```python
from build123d import *

# Parameters (mm, degrees)
SKETCH_1_W          = 17
SKETCH_1_H          = 11.5
EXTRUDE_1_DEPTH     = 1.5
SKETCH_2_R          = 4
EXTRUDE_2_DEPTH     = 3
SKETCH_3_R          = 2
CUT_EXTRUDE_1_DEPTH = 0.2
SKETCH_4_R          = 0.5
SKETCH_4_R_2        = 1.5
CUT_EXTRUDE_2_DEPTH = 11.69170239


with BuildPart() as part:
    # Эскиз1 → Бобышка-Вытянуть1 (new body)
    with BuildSketch(Plane(origin=(0, 0, 0), x_dir=(1, 0, 0), z_dir=(0, 1, 0))):
        Rectangle(SKETCH_1_W, SKETCH_1_H)
    extrude(amount=EXTRUDE_1_DEPTH)

    # Эскиз2 → Бобышка-Вытянуть2 (add)
    with BuildSketch(Plane(origin=(0, 1.5, 0), x_dir=(1, 0, 0), z_dir=(0, 1, 0))):
        with Locations(Location((0, 0, 0), (0, 0, 270))):
            Circle(SKETCH_2_R)
    extrude(amount=EXTRUDE_2_DEPTH)

    # Эскиз3 → Вырез-Вытянуть1 (cut)
    with BuildSketch(Plane(origin=(0, 4.5, 0), x_dir=(1, 0, 0), z_dir=(0, 1, 0))):
        with Locations(Location((0, 0, 0), (0, 0, 270))):
            Circle(SKETCH_3_R)
    extrude(amount=-CUT_EXTRUDE_1_DEPTH, mode=Mode.SUBTRACT)

    # Эскиз4 → Вырез-Вытянуть2 (cut, through all)
    with BuildSketch(Plane(origin=(0, 1.5, 0), x_dir=(1, 0, 0), z_dir=(0, 1, 0))):
        with Locations(Location((6.5, 3.81, 0), (0, 0, 270))):
            Circle(SKETCH_4_R)
        with Locations(Location((6.5, 1.27, 0), (0, 0, 270))):
            Circle(SKETCH_4_R)
        with Locations(Location((6.5, -1.27, 0), (0, 0, 270))):
            Circle(SKETCH_4_R)
        with Locations(Location((6.5, -3.81, 0), (0, 0, 270))):
            Circle(SKETCH_4_R)
        with Locations(Location((-6.43732089, 3, 0), (0, 0, 270))):
            Circle(SKETCH_4_R_2)
        with Locations(Location((-6.43732089, -3, 0), (0, 0, 270))):
            Circle(SKETCH_4_R_2)
    extrude(amount=-CUT_EXTRUDE_2_DEPTH, mode=Mode.SUBTRACT)


solid = part.part
```
Check sheet for the modelled part. Datum: model origin and axes. Units: mm. A direction names the side the tool comes from. Give positions to 0.01 mm unless a question says otherwise; leave off trailing zeros. Write each loop counter-clockwise with the first axis right and the second up, starting at its lowest first coordinate (ties: lowest second). Pieces come first, ordered by that corner, then holes. Notation, with made-up numbers: (-38, 66) - (13, 66) arc R20 cw to (13, 73) - close; hole circle Ø8 at (74, 80). An arc over 180 degrees is marked (long way). Answer as a JSON object with one key per item and string values. Group by question number.
1) Depth check by flat-ended pin: P1, Ø5, axis at x = -6.44, z = -3, coming from the +Y side; P2, Ø1.5, axis at y = 2.5, z = 2, coming from the -X side. Enter the tip coordinate at first touch or a pass-through.
2) Thickness scan on probe 1 along X at (y, z) = (0.7, 3); probe 2 along X at (y, z) = (0.95, 1.27); probe 3 along Z at (x, y) = (-7.25, 1.05). Record the ranges inside material, lowest first. Write a range as from..to.
3) Release check for a two-part mould opening along X. For faces 3 (the face through (0, 1, 5.75)), 4 (the face through (0, 4.3, 0)), 5 (the face through (6.056, 0.76, -1.039)), 6 (the face through (8.5, 1, 0)) record: pulls with the +X half, pulls with the -X half, needs draft (parallel to the pull), parting line crosses it, or undercut.
4) Sectioned sample at D-D (y = 3.95). Record the cut outline in (x, z).
5) Sectioned sample at C-C (x = 0). Record the cut outline in (y, z), then the cut area to 4 significant figures.
6) Sectioned sample at B-B (x = -7.5). Record the cut outline in (y, z), then the cut area to 3 significant figures.
7) Sectioned sample at A-A (z = -1). Record the cut outline in (x, y), then the cut area to 3 significant figures.
8) Access from +Z, -Z, +X, -X, +Y, -Y to the whole of each face (thin tool, end or side, straight path). Record for faces 1 (the face through (-4.95, 0.76, -3.2)), 2 (the face through (-3.905, 2.979, -0.867)).
Geometry results:
{
 "1": {"P1": "stops at y = 1.5", "P2": "stops at x = -3.8"},
 "2": {"probe 1": "x = -8.5..-7.94, -4.94..8.5", "probe 2": "x = -8.5..6, 7..8.5", "probe 3": "z = -5.75..-4.26, -1.74..1.74, 4.26..5.75"},
 "3": {"face 3": "needs draft", "face 4": "undercut", "face 5": "undercut", "face 6": "pulls with the +X half"},
 "4": {"outline": "circle Ø8 at (0, 0)"},
 "5": {"outline": "(0, -5.75) - (1.5, -5.75) - (1.5, -4) - (4.5, -4) - (4.5, -2) - (4.3, -2) - (4.3, 2) - (4.5, 2) - (4.5, 4) - (1.5, 4) - (1.5, 5.75) - (0, 5.75) - close", "area": "40.45 mm^2"},
 "6": {"outline": "(0, -5.75) - (1.5, -5.75) - (1.5, -4.06) - (0, -4.06) - close; (0, -1.94) - (1.5, -1.94) - (1.5, 1.94) - (0, 1.94) - close; (0, 4.06) - (1.5, 4.06) - (1.5, 5.75) - (0, 5.75) - close", "area": "10.9 mm^2"},
 "7": {"outline": "(-8.5, 0) - (6.08, 0) - (6.08, 1.5) - (3.87, 1.5) - (3.87, 4.5) - (1.73, 4.5) - (1.73, 4.3) - (-1.73, 4.3) - (-1.73, 4.5) - (-3.87, 4.5) - (-3.87, 1.5) - (-8.5, 1.5) - close; (6.92, 0) - (8.5, 0) - (8.5, 1.5) - (6.92, 1.5) - close", "area": "46.8 mm^2"},
 "8": {"face 1": "+Y, -Y", "face 2": "+Y"}
}
